Check sheet for the modelled part. Datum: model origin and axes. Units: mm. A direction names the side the tool comes from. Coordinates: 2 decimals unless noted, no trailing zeros. Order: outer loops, then holes, each group sorted by start corner. A loop starts at its lowest first (then second) coordinate and runs counter-clockwise, first axis right, second up.
from build123d import *

# Parameters (mm, degrees)
SKETCH1_R           = 4
BOSS_EXTRUDE1_DEPTH = 28
CUT_EXTRUDE1_DEPTH  = 11.5
SKETCH3_R           = 1
CUT_EXTRUDE2_DEPTH  = 4
FILLET1_R           = 0.5


with BuildPart() as part:
    # Sketch1 → Boss-Extrude1 (new body)
    with BuildSketch(Plane.XY):
        Circle(SKETCH1_R)
    extrude(amount=BOSS_EXTRUDE1_DEPTH)

    # Sketch2 → Cut-Extrude1 (cut)
    with BuildSketch(Plane.XY.offset(28)):
        with BuildLine():
            Line((-3, 2.645751311), (3, 2.645751311))
            ThreePointArc((3, 2.645751311), (0, 4), (-3, 2.645751311))
        make_face()
    extrude(amount=-CUT_EXTRUDE1_DEPTH, mode=Mode.SUBTRACT)

    # Sketch3 → Cut-Extrude2 (cut)
    with BuildSketch(Plane.XY.offset(28)):
        Circle(SKETCH3_R)
    extrude(amount=-CUT_EXTRUDE2_DEPTH, mode=Mode.SUBTRACT)

    # Fillet1
    fillet1_edges = [part.edges().sort_by_distance(p)[0] for p in [
        (-1, 0, 28),
        (-1.414213562, -3.741657387, 28),
        (0, 4, 16.5),
        (0, 2.645751311, 28),
    ]]
    fillet(fillet1_edges, radius=FILLET1_R)


solid = part.part
(1) Cross-section at A-A (x = 0). Enter the section's corners in (y, z), and give its area (3 significant figures).
Filled in:
outline: (-4, 0) - (4, 0) - (4, 16) arc R0.5 ccw to (3.5, 16.5) - (2.65, 16.5) - (2.65, 27.5) arc R0.5 ccw to (2.15, 28) - (1.5, 28) arc R0.5 ccw to (1, 27.5) - (1, 24) - (-1, 24) - (-1, 27.5) arc R0.5 ccw to (-1.5, 28) - (-3.5, 28) arc R0.5 ccw to (-4, 27.5) - close
area: 200 mm2
(2) Tool access check on faces 1 (the flat face through (0, -2, 28)), 2 (the flat face through (0, 0, 24)). Record the directions out of +Z, -Z, +X, -X, +Y, -Y that give a thin tool (end or side, any length) a straight path to the whole face; none if there is none.
Filled in:
face 1: +Z, +X, -X, +Y, -Y
face 2: +Z
(3) Thickness scan on probe 1 along Y at (x, z) = (0, 26.3); probe 2 along Z at (x, y) = (0.25, -0.75); probe 3 along Y at (x, z) = (-0.25, 14.25). Record the ranges inside material, lowest first.
Filled in:
probe 1: y = -4 to -1, 1 to 2.65
probe 2: z = 0 to 24
probe 3: y = -3.99 to 3.99
(4) Go/stop test with a flat-tipped pin: P1, Ø1, axis at x = 0, y = 0, coming from the +Z side. Record where the tip stops, or that it passes through.
Filled in:
P1: stops at z = 24
(5) Cross-section at C-C (z = 6.75). Enter the section's corners in (x, y).
Filled in:
outline: circle Ø8 at (0, 0)
(6) Cross-section at B-B (z = 25.75). Enter the section's corners in (x, y), and give its area (3 significant figures).
Filled in:
outline: (-3, 2.65) arc R4 ccw (long way) to (3, 2.65) - close; hole circle Ø2 at (0, 0)
area: 41.5 mm2
(7) Release check for a two-part mould opening along Y. For faces 3 (the flat face through (0, 3, 16.5)), 4 (the flat face through (0, 2.646, 22)), 5 (the cylindrical face through (0, -1, 26)) record: +Y half, -Y half, draft (parallel to the pull), parting line (faces both ways), or undercut.
Filled in:
face 3: draft
face 4: +Y half
face 5: undercut
